```python
from build123d import *

# Parameters (mm, degrees)
SKETCH1_R           = 2
BOSS_EXTRUDE1_DEPTH = 10


with BuildPart() as part:
    # Sketch1 → Boss-Extrude1 (new body)
    with BuildSketch(Plane.XY):
        with BuildLine():
            Line((0, 0), (230, 0))
            Line((230, 0), (230, 37.5))
            ThreePointArc((230, 37.5), (220, 52.5), (230, 67.5))
            Line((230, 67.5), (230, 105))
            Line((230, 105), (0, 105))
            Line((0, 105), (0, 67.5))
            ThreePointArc((0, 67.5), (10, 52.5), (0, 37.5))
            Line((0, 37.5), (0, 0))
        make_face()
        with Locations((208, 52.5)):
            Circle(SKETCH1_R, mode=Mode.SUBTRACT)
        with Locations(Location((22, 52.5, 0), (0, 0, 180))):
            Circle(SKETCH1_R, mode=Mode.SUBTRACT)
    extrude(amount=BOSS_EXTRUDE1_DEPTH)


solid = part.part
```
Input: part model. Units: mm. Frame: model coordinates. Round coordinates to 2 decimals unless told otherwise and drop trailing zeros. Loops run counter-clockwise (first coordinate to the right, second up) from the corner with the lowest first, then second, coordinate; pieces in that order, holes last. Notation, with made-up numbers: M 54.5,-38.75 L 67.5,-38.75 A16 ccw 67.5,-26.75 Z; hole C 37.5,-13 d6. An arc over 180 degrees is marked long. Answer in a Markdown table with one row per item. Add a question column.
1. Ray query, probe 1 along Y at (x, z) = (22, 2.75); probe 2 along X at (y, z) = (64, 4); probe 3 along X at (y, z) = (59, 7). Return the intervals inside material, ascending.
2. Section B-B (y = 47). Output: boundary loops of the cut face in (x, z), and give its area (3 significant figures).
3. Mould query, pull axis Y, two halves, no side actions, for faces 1 (the face through (230, 86, 5)), 2 (the face through (22.434, 54.452, 4.93)), 3 (the face through (206.002, 52.588, 4.93)), 4 (the face through (113, 0, 5)). Classes: released by +Y, released by -Y, zero draft, split by the parting line, or undercut.
4. Section A-A (z = 7.5). Output: boundary loops of the cut face in (x, y), and give its area (3 significant figures).
Values follow:
| question | item | result |
|---|---|---|
| 1 | probe 1 | 0 to 50.5, 54.5 to 105 |
| 1 | probe 2 | 5.23 to 224.77 |
| 1 | probe 3 | 8.64 to 221.36 |
| 2 | outline | M 9.04,0 L 220.96,0 L 220.96,10 L 9.04,10 Z |
| 2 | area | 2,120 mm^2 |
| 3 | face 1 | zero draft |
| 3 | face 2 | undercut |
| 3 | face 3 | undercut |
| 3 | face 4 | released by -Y |
| 4 | outline | M 0,0 L 230,0 L 230,37.5 A16.25 cw 230,67.5 L 230,105 L 0,105 L 0,67.5 A16.25 cw 0,37.5 Z; hole C 22,52.5 d4; hole C 208,52.5 d4 |
| 4 | area | 23,700 mm^2 |
